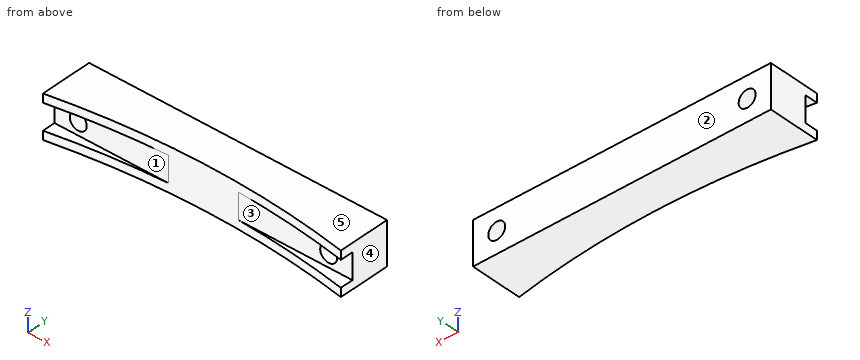
from build123d import *

# Parameters (mm, degrees)
BOSS_EXTRUDE1_DEPTH = 12.7
SKETCH2_R           = 2.5
CUT_EXTRUDE1_DEPTH  = 16.24
SKETCH3_W           = 7.62
SKETCH3_H           = 3.81
CUT_EXTRUDE2_DEPTH  = 88.8100001


with BuildPart() as part:
    # Sketch1 → Boss-Extrude1 (new body)
    with BuildSketch(Plane.XY):
        with BuildLine():
            Line((-43.905, 0), (43.905, 0))
            Line((43.905, 0), (43.905, -15.24))
            ThreePointArc((43.905, -15.24), (0, -11.212082165), (-43.905, -15.24))
            Line((-43.905, -15.24), (-43.905, 0))
        make_face()
    extrude(amount=BOSS_EXTRUDE1_DEPTH)

    # Sketch2 → Cut-Extrude1 (cut, through all)
    with BuildSketch(Plane(origin=(0, 0, 0), x_dir=(1, 0, 0), z_dir=(0, 1, 0))):
        with Locations((-36.905, -6.35)):
            Circle(SKETCH2_R)
        with Locations((36.905, -6.35)):
            Circle(SKETCH2_R)
    extrude(amount=-CUT_EXTRUDE1_DEPTH, mode=Mode.SUBTRACT)

    # Sketch3 → Cut-Extrude2 (cut, through all)
    with BuildSketch(Plane(origin=(43.905, 0, 0), x_dir=(0, 0, -1), z_dir=(1, 0, 0))):
        with Locations((-6.35, -13.335)):
            Rectangle(SKETCH3_W, SKETCH3_H)
    extrude(amount=-CUT_EXTRUDE2_DEPTH, mode=Mode.SUBTRACT)


solid = part.part
CAD build for the part. Positions are in the model's coordinates, mm. Face numbers are marked on the shaded views. A direction names the side the tool comes from. Coordinates: 2 decimals unless noted, no trailing zeros. Loops run counter-clockwise (first coordinate to the right, second up) from the corner with the lowest first, then second, coordinate; pieces in that order, holes last. Notation, with made-up numbers: (79, 78) - (113, 78) arc R38 cw to (113, 117) - close; hole circle Ø1 at (67, -6.5). An arc over 180 degrees is marked (long way). Write item = value, one per line. Start each with the question number.
Q1. Cut at B-B, the plane y = -12.5. List the corners of the cut face in (x, z) (3 decimals).
Q2. Flat gauge pins, fed straight in: pin 1 Ø6 at (x, z) = (23.5, 1.5) entering from +Y; pin 2 Ø5 at (x, z) = (-8.5, 10.5) entering from -Y; pin 3 Ø4 at (x, z) = (34.5, 5.5) entering from -Y; pin 4 Ø5 at (x, z) = (-1.5, 8.5) entering from -Y. Where does each tip first touch, or does it go through?
Q3. Drill centre lines: L1, parallel to X at y = -6.5, z = 6.35 (3 decimals); L2, parallel to Z at x = 18.5, y = -11.75; L3, parallel to X at y = -3.5, z = 5.25 (3 decimals). Where is each one in solid material? Low to high.
Q4. Cut at D-D, the plane y = -4.25. List the corners of the cut face in (x, z) (3 decimals), then the cut area to 3 significant figures.
Q5. Pull direction Z, two halves, no side cores. Call the marked faces 3, 4 and 5: pulls with the +Z half, pulls with the -Z half, needs draft (parallel to the pull), parting line crosses it, or undercut.
Q6. Cut at A-A, the plane z = 6.35. List the corners of the cut face in (x, y) (3 decimals).
Q7. Cut at C-C, the plane x = 37. List the corners of the cut face in (y, z), then the cut area to 3 significant figures.
Q8. Which spindle directions (+Z, -Z, +X, -X, +Y, -Y) get a long thin tool onto all of the face, cutting with end or side? Do the marked faces 1 and 2. Say none if no direction does.
Computed:
q1.outline = (-43.905, 0) - (-24.898, 0) - (-24.898, 2.54) - (-43.905, 2.54) - close; (-43.905, 10.16) - (-24.898, 10.16) - (-24.898, 12.7) - (-43.905, 12.7) - close; (24.898, 0) - (43.905, 0) - (43.905, 2.54) - (24.898, 2.54) - close; (24.898, 10.16) - (43.905, 10.16) - (43.905, 12.7) - (24.898, 12.7) - close
q2.pin_1 = 0
q2.pin_2 = -11.46
q2.pin_3 = -11.43
q2.pin_4 = -11.25
q3.L1 = -43.905 to -39.405, -34.405 to 34.405, 39.405 to 43.905
q3.L2 = 0 to 2.54, 10.16 to 12.7
q3.L3 = -43.905 to -39.15, -34.66 to 34.66, 39.15 to 43.905
q4.outline = (-43.905, 0) - (43.905, 0) - (43.905, 12.7) - (-43.905, 12.7) - close; hole circle Ø5 at (-36.905, 6.35); hole circle Ø5 at (36.905, 6.35)
q4.area = 1,080 mm²
q5.face_3 = undercut
q5.face_4 = needs draft
q5.face_5 = pulls with the +Z half
q6.outline = (-43.905, -11.43) - (-39.405, -11.43) - (-39.405, 0) - (-43.905, 0) - close; (-34.405, -11.43) - (-10.253, -11.43) arc R241.3 cw to (10.253, -11.43) - (34.405, -11.43) - (34.405, 0) - (-34.405, 0) - close; (39.405, -11.43) - (43.905, -11.43) - (43.905, 0) - (39.405, 0) - close
q7.outline = (-14.07, 0) - (0, 0) - (0, 3.85) - (-11.43, 3.85) - (-11.43, 2.54) - (-14.07, 2.54) - close; (-14.07, 10.16) - (-11.43, 10.16) - (-11.43, 8.85) - (0, 8.85) - (0, 12.7) - (-14.07, 12.7) - close
q7.area = 101 mm²
q8.face_1 = +X, -X, -Y
q8.face_2 = +Z, -Z, +X, -X, +Y
